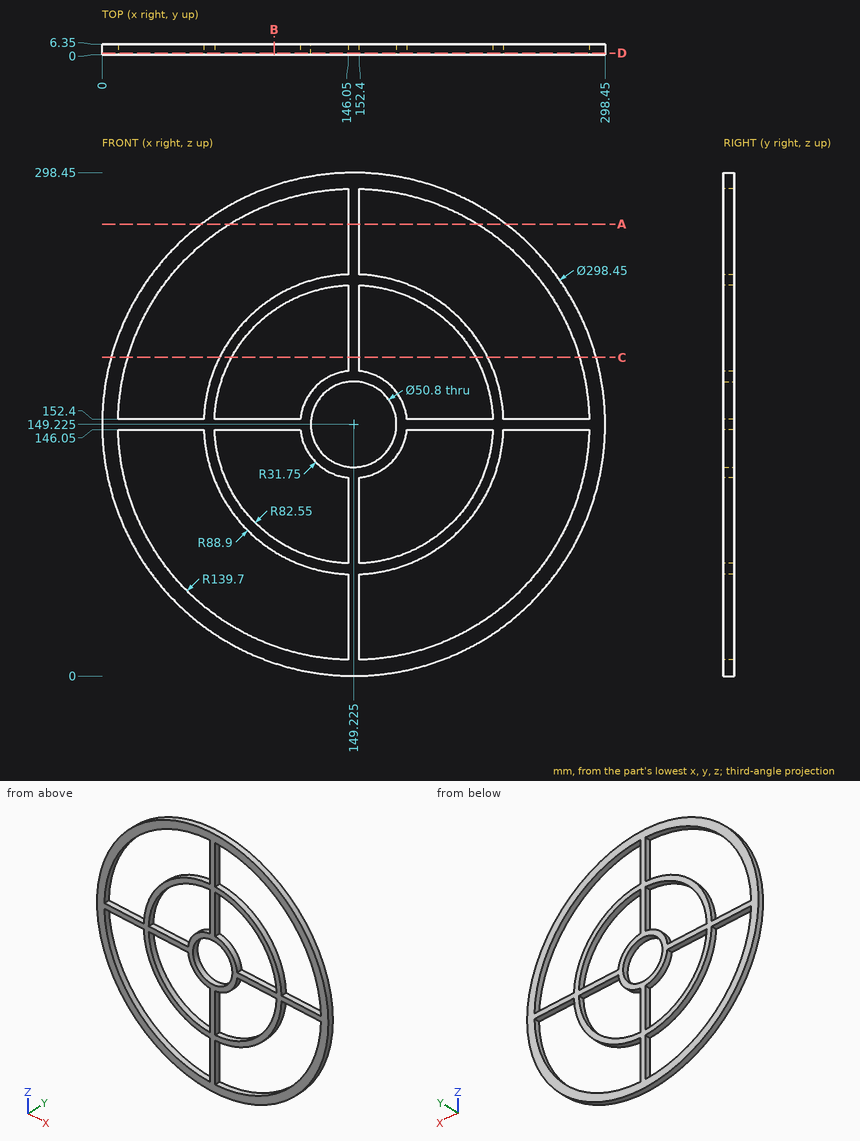
Geometry: see drawing. Coordinates: mm, zero at the bounding-box minimum. Round coordinates to 2 decimals unless told otherwise and drop trailing zeros. Loops run counter-clockwise (first coordinate to the right, second up) from the corner with the lowest first, then second, coordinate; pieces in that order, holes last. Notation, with made-up numbers: (41.25, 41.5) -> (57.25, 41.5) arc R14 ccw to (57.25, 45.5) -> close; hole circle Ø1 at (30, 40). An arc over 180 degrees is marked (long way). Use one line per item in the form item = value. Start each with the question number.
Item 1: Section query A-A on z = 268. Return the cut outline in (x, y), then the cut area to 3 significant figures.
Item 2: Section query D-D on y = 1. Count the separate pieces of the cut face and the enclosed holes in it, then the cut area to 3 significant figures.
Item 3: Section query B-B on x = 102. Return the cut outline in (y, z), then the cut area to 3 significant figures.
Item 4: Material intervals for L1, parallel to Z at x = 20.5, y = 0.5; L2, parallel to X at y = 3, z = 175.5; L3, parallel to Z at x = 97.5, y = 5.5, sorted ascending. Write a range as from..to.
Item 5: Section query C-C on z = 189. Return the cut outline in (x, y), then the cut area to 3 significant figures.
Item 6: Contact query for flat-ended pins moving along their axis: pin 1 Ø1.5 at (y, z) = (2.5, 90.5) entering from +X; pin 2 Ø1 at (x, y) = (200.5, 2.5) entering from +Z; pin 3 Ø1.9 at (y, z) = (3.5, 101) entering from +X; pin 4 Ø2 at (x, z) = (263.5, 247.5) entering from +Y. Output: stop coordinate, or through.
Ans:
q1.outline = (58.89, 0) -> (75.68, 0) -> (75.68, 6.35) -> (58.89, 6.35) -> close; (146.05, 0) -> (152.4, 0) -> (152.4, 6.35) -> (146.05, 6.35) -> close; (222.77, 0) -> (239.56, 0) -> (239.56, 6.35) -> (222.77, 6.35) -> close
q1.area = 254 mm^2
q2.separate_pieces = 1
q2.enclosed_holes = 9
q2.area = 15,800 mm^2
q3.outline = (0, 7.67) -> (6.35, 7.67) -> (6.35, 17.75) -> (0, 17.75) -> close; (0, 73.91) -> (6.35, 73.91) -> (6.35, 81.52) -> (0, 81.52) -> close; (0, 146.05) -> (6.35, 146.05) -> (6.35, 152.4) -> (0, 152.4) -> close; (0, 216.93) -> (6.35, 216.93) -> (6.35, 224.54) -> (0, 224.54) -> close; (0, 280.7) -> (6.35, 280.7) -> (6.35, 290.78) -> (0, 290.78) -> close
q3.area = 265 mm^2
q4.L1 = 73.74..94.95, 146.05..152.4, 203.5..224.71
q4.L2 = 2.33..12.02, 64.3..70.97, 131.4..167.05, 227.48..234.15, 286.43..296.12
q4.L3 = 9.25..19.45, 76.92..84.89, 146.05..152.4, 213.56..221.53, 279..289.2
q5.outline = (5.4, 0) -> (15.31, 0) -> (15.31, 6.35) -> (5.4, 6.35) -> close; (69.72, 0) -> (76.89, 0) -> (76.89, 6.35) -> (69.72, 6.35) -> close; (146.05, 0) -> (152.4, 0) -> (152.4, 6.35) -> (146.05, 6.35) -> close; (221.56, 0) -> (228.73, 0) -> (228.73, 6.35) -> (221.56, 6.35) -> close; (283.14, 0) -> (293.05, 0) -> (293.05, 6.35) -> (283.14, 6.35) -> close
q5.area = 257 mm^2
q6.pin_1 = 286.73
q6.pin_2 = 289.55
q6.pin_3 = 290.76
q6.pin_4 = through
